from build123d import *

# Parameters (mm, degrees)
SKETCH1_R             = 50
SKETCH1_R_2           = 3
SKETCH1_W             = 21
SKETCH1_H             = 25
BOSS_EXTRUDE1_DEPTH   = 6.35
M3X0_5_TAPPED_HOLE1_D = 2.5


with BuildPart() as part:
    # Sketch1 → Boss-Extrude1 (new body)
    with BuildSketch(Plane(origin=(0, 0, 0), x_dir=(1, 0, 0), z_dir=(0, 1, 0))):
        with Locations(Location((0, 0, 0), (0, 0, 270))):
            Circle(SKETCH1_R)
        with Locations(Location((22, 22, 0), (0, 0, 270))):
            Circle(SKETCH1_R_2, mode=Mode.SUBTRACT)
        with Locations(Location((-22, 22, 0), (0, 0, 270))):
            Circle(SKETCH1_R_2, mode=Mode.SUBTRACT)
        with Locations(Location((-22, -22, 0), (0, 0, 270))):
            Circle(SKETCH1_R_2, mode=Mode.SUBTRACT)
        with Locations(Location((22, -22, 0), (0, 0, 270))):
            Circle(SKETCH1_R_2, mode=Mode.SUBTRACT)
        with Locations((0, 5.5)):
            Rectangle(SKETCH1_W, SKETCH1_H, mode=Mode.SUBTRACT)
    extrude(amount=BOSS_EXTRUDE1_DEPTH)

    # M3x0.5 Tapped Hole1 (through all)
    with Locations(Plane(origin=(0, 0, 0), x_dir=(-1, 0, 0), z_dir=(0, -1, 0))):
        with Locations((21.59, 8.89), (-24.13, 8.89), (-24.13, -8.89), (21.59, -8.89), (31.75, 8.89), (-34.29, 8.89), (31.75, -8.89), (-34.29, -8.89)):
            Hole(M3X0_5_TAPPED_HOLE1_D / 2)


solid = part.part
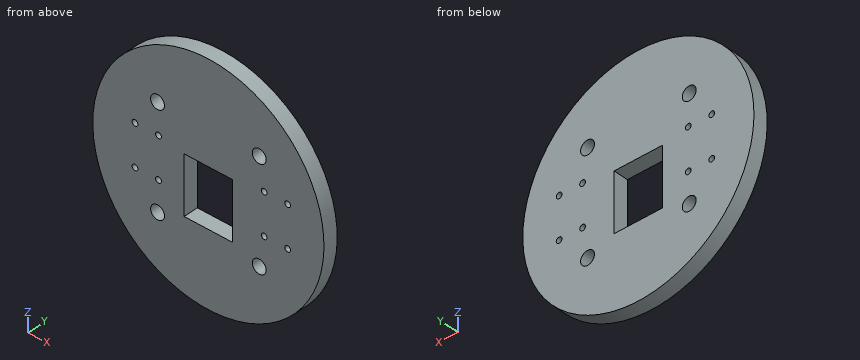
Model file for the job. Use its own axes, mm. Give positions to 0.01 mm unless a question says otherwise; leave off trailing zeros. Order: outer loops, then holes, each group sorted by start corner. A loop starts at its lowest first (then second) coordinate and runs counter-clockwise, first axis right, second up. Notation, with made-up numbers: (8.25, 35.25) - (64.25, 35.25) arc R13 ccw to (64.25, 51.25) - close; hole circle Ø5 at (47.25, 72.5). An arc over 180 degrees is marked (long way). Write item = value, one per line. Start each with the question number.
1. Cut at D-D, the plane x = -14. List the corners of the cut face in (y, z).
2. Cut at C-C, the plane z = 0.5. List the corners of the cut face in (x, y).
3. Cut at B-B, the plane z = 23. List the corners of the cut face in (x, y), and give its area (3 significant figures).
4. Cut at A-A, the plane y = 3.75. State how many separate pieces and enclosed holes the cut face has, and give its area (3 significant figures).
5. Probe line 1 along X through (y, z) = (4, -8.89); line 2 along Z through (x, y) = (34.29, 5.25); line 3 along Z through (x, y) = (-23, 4.5). List the from-to ranges inside material, lowest first.
6. Drop flat-ended pins along their axis: P1, Ø1, axis at x = -5.5, y = 5.5, coming from the +Z side; P2, Ø1, axis at x = -34.5, z = 6.5, coming from the -Y side; P3, Ø1.9, axis at y = 2, z = -10.5, coming from the -X side; P4, Ø1, axis at x = 40, y = 1.5, coming from the +Z side. Give the stop position or say it passes through.
Taken from the geometry:
q1.outline = (0, -48) - (6.35, -48) - (6.35, 48) - (0, 48) - close
q2.outline = (-50, 0) - (-10.5, 0) - (-10.5, 6.35) - (-50, 6.35) - close; (10.5, 0) - (50, 0) - (50, 6.35) - (10.5, 6.35) - close
q3.outline = (-44.4, 0) - (-24.83, 0) - (-24.83, 6.35) - (-44.4, 6.35) - close; (-19.17, 0) - (19.17, 0) - (19.17, 6.35) - (-19.17, 6.35) - close; (24.83, 0) - (44.4, 0) - (44.4, 6.35) - (24.83, 6.35) - close
q3.area = 492 mm²
q4.separate_pieces = 1
q4.enclosed_holes = 13
q4.area = 7,180 mm²
q5.line_1 = -49.2 to -33, -30.5 to -22.84, -20.34 to -10.5, 10.5 to 22.88, 25.38 to 33.04, 35.54 to 49.2
q5.line_2 = -36.39 to -10.14, -7.64 to 7.64, 10.14 to 36.39
q5.line_3 = -44.4 to -24.83, -19.17 to 19.17, 24.83 to 44.4
q6.P1 = 49.75
q6.P2 = 0
q6.P3 = -49.08
q6.P4 = 30.66
